Input: part model. Units: mm. Frame: model coordinates. A direction names the side the tool comes from. Round coordinates to 2 decimals unless told otherwise and drop trailing zeros. Loops run counter-clockwise (first coordinate to the right, second up) from the corner with the lowest first, then second, coordinate; pieces in that order, holes last. Notation, with made-up numbers: (87.25, 82) - (143.25, 82) arc R20 ccw to (143.25, 108) - close; hole circle Ø3 at (72, 65). An arc over 180 degrees is marked (long way). Write each question's results on one line, items separated by ' | '.
from build123d import *

# Parameters (mm, degrees)
SKETCH1_R           = 79.375
BOSS_EXTRUDE1_DEPTH = 25.4
SKETCH2_R           = 28.575
BOSS_EXTRUDE2_DEPTH = 3.175
SKETCH3_R           = 9.525
CUT_EXTRUDE1_DEPTH  = 19.05


with BuildPart() as part:
    # Sketch1 → Boss-Extrude1 (new body)
    with BuildSketch(Plane(origin=(0, 0, 0), x_dir=(1, 0, 0), z_dir=(0, 1, 0))):
        with Locations(Location((0, 0, 0), (0, 0, 270))):
            Circle(SKETCH1_R)
        with BuildLine():
            ThreePointArc((12.296722124, 3.175), (11.733270063, 4.860079591), (10.940159631, 6.45003157))
            Line((10.940159631, 6.45003157), (56.079808271, 51.589680211))
            ThreePointArc((56.079808271, 51.589680211), (70.399620377, 29.160477546), (76.133825433, 3.175))
            Line((76.133825433, 3.175), (12.296722124, 3.175))
        make_face(mode=Mode.SUBTRACT)
        with BuildLine():
            Line((51.589680211, 56.079808271), (6.45003157, 10.940159631))
            ThreePointArc((6.45003157, 10.940159631), (4.860079591, 11.733270063), (3.175, 12.296722124))
            Line((3.175, 12.296722124), (3.175, 76.133825433))
            ThreePointArc((3.175, 76.133825433), (29.160477546, 70.399620377), (51.589680211, 56.079808271))
        make_face(mode=Mode.SUBTRACT)
        with BuildLine():
            Line((-3.175, 76.133825433), (-3.175, 12.296722124))
            ThreePointArc((-3.175, 12.296722124), (-4.860079591, 11.733270063), (-6.45003157, 10.940159631))
            Line((-6.45003157, 10.940159631), (-51.589680211, 56.079808271))
            ThreePointArc((-51.589680211, 56.079808271), (-29.160477546, 70.399620377), (-3.175, 76.133825433))
        make_face(mode=Mode.SUBTRACT)
        with BuildLine():
            Line((-56.079808271, 51.589680211), (-10.940159631, 6.45003157))
            ThreePointArc((-10.940159631, 6.45003157), (-11.733270063, 4.860079591), (-12.296722124, 3.175))
            Line((-12.296722124, 3.175), (-76.133825433, 3.175))
            ThreePointArc((-76.133825433, 3.175), (-70.399620377, 29.160477546), (-56.079808271, 51.589680211))
        make_face(mode=Mode.SUBTRACT)
        with BuildLine():
            Line((-76.133825433, -3.175), (-12.296722124, -3.175))
            ThreePointArc((-12.296722124, -3.175), (-11.733270063, -4.860079591), (-10.940159631, -6.45003157))
            Line((-10.940159631, -6.45003157), (-56.079808271, -51.589680211))
            ThreePointArc((-56.079808271, -51.589680211), (-70.399620377, -29.160477546), (-76.133825433, -3.175))
        make_face(mode=Mode.SUBTRACT)
        with BuildLine():
            Line((-51.589680211, -56.079808271), (-6.45003157, -10.940159631))
            ThreePointArc((-6.45003157, -10.940159631), (-4.860079591, -11.733270063), (-3.175, -12.296722124))
            Line((-3.175, -12.296722124), (-3.175, -76.133825433))
            ThreePointArc((-3.175, -76.133825433), (-29.160477546, -70.399620377), (-51.589680211, -56.079808271))
        make_face(mode=Mode.SUBTRACT)
        with BuildLine():
            Line((3.175, -76.133825433), (3.175, -12.296722124))
            ThreePointArc((3.175, -12.296722124), (4.860079591, -11.733270063), (6.45003157, -10.940159631))
            Line((6.45003157, -10.940159631), (51.589680211, -56.079808271))
            ThreePointArc((51.589680211, -56.079808271), (29.160477546, -70.399620377), (3.175, -76.133825433))
        make_face(mode=Mode.SUBTRACT)
        with BuildLine():
            Line((56.079808271, -51.589680211), (10.940159631, -6.45003157))
            ThreePointArc((10.940159631, -6.45003157), (11.733270063, -4.860079591), (12.296722124, -3.175))
            Line((12.296722124, -3.175), (76.133825433, -3.175))
            ThreePointArc((76.133825433, -3.175), (70.399620377, -29.160477546), (56.079808271, -51.589680211))
        make_face(mode=Mode.SUBTRACT)
    extrude(amount=BOSS_EXTRUDE1_DEPTH)

    # Sketch2 → Boss-Extrude2 (add)
    with BuildSketch(Plane.XZ):
        Circle(SKETCH2_R)
    extrude(amount=-BOSS_EXTRUDE2_DEPTH)

    # Sketch3 → Cut-Extrude1 (cut)
    with BuildSketch(Plane.XZ):
        with Locations(Location((0, 0, 0), (0, 0, 270))):
            Circle(SKETCH3_R)
    extrude(amount=-CUT_EXTRUDE1_DEPTH, mode=Mode.SUBTRACT)


solid = part.part
1. Mould query, pull axis Z, two halves, no side actions, for faces 1 (the flat face through (9, 3.175, -20)), 2 (the flat face through (-17, 0, -1)). Classes: pulls with the +Z half, pulls with the -Z half, needs draft (parallel to the pull), parting line crosses it, or undercut.
Answer:
face 1: undercut | face 2: needs draft
2. Section query C-C, the plane x = -32. Output: boundary loops of the cut face in (y, z) (3 decimals), plus the area to 3 significant figures.
Answer:
outline: (0, -72.639) - (25.4, -72.639) - (25.4, -69.155) - (0, -69.155) - close; (0, -36.49) - (25.4, -36.49) - (25.4, -27.51) - (0, -27.51) - close; (0, -3.175) - (25.4, -3.175) - (25.4, 3.175) - (0, 3.175) - close; (0, 27.51) - (25.4, 27.51) - (25.4, 36.49) - (0, 36.49) - close; (0, 69.155) - (25.4, 69.155) - (25.4, 72.639) - (0, 72.639) - close | area: 794 mm^2
3. Section query B-B, the plane z = 48. Output: boundary loops of the cut face in (x, y) (3 decimals), plus the area to 3 significant figures.
Answer:
outline: (-63.217, 0) - (-59.181, 0) - (-59.181, 25.4) - (-63.217, 25.4) - close; (-52.49, 0) - (-43.51, 0) - (-43.51, 25.4) - (-52.49, 25.4) - close; (-3.175, 0) - (3.175, 0) - (3.175, 25.4) - (-3.175, 25.4) - close; (43.51, 0) - (52.49, 0) - (52.49, 25.4) - (43.51, 25.4) - close; (59.181, 0) - (63.217, 0) - (63.217, 25.4) - (59.181, 25.4) - close | area: 822 mm^2
4. Line query: line 1 (Z direction, x = 5.5, y = 20.75); line 2 (X direction, y = 7.25, z = 0) (3 decimals); line 3 (X direction, y = 19.5, z = 55) (3 decimals). Output: solid intervals per line, ascending. Write a range as [from, to].
Answer:
line 1: [-79.18, -76], [-11.45, 11.45], [76, 79.18] | line 2: [-79.375, -9.525], [9.525, 79.375] | line 3: [-57.231, -50.51], [-3.175, 3.175], [50.51, 57.231]
5. Set-up query: faces 3 (the cylindrical face through (-11.039, 1.565, -26.357)), 4 (the cylindrical face through (-5.796, 9.392, 7.559)), 5 (the flat face through (33.83, 12.52, 29.34)). Return all of +Z, -Z, +X, -X, +Y, -Y with unobstructed straight access to the full face (end or side cutting, diameter ignored); none if empty.
Answer:
face 3: +Y, -Y | face 4: -Y | face 5: +Y
6. Contact query for flat-ended pins moving along their axis: pin 1 (1.5 mm diameter, centred on x = -41.5, y = 20, fed in from -Z); pin 2 (7.5 mm diameter, centred on y = 13.5, z = 48, fed in from +X); pin 3 (10 mm diameter, centred on x = 13.5, z = -34.5, fed in from +Y); pin 4 (4 mm diameter, centred on y = 8, z = 13, fed in from -X). Output: stop coordinate, or through.
Answer:
pin 1: z = -68.12 | pin 2: x = 65.9 | pin 3: through | pin 4: x = -78.61
7. Section query A-A, the plane y = 11. Count the separate pieces of the cut face and the enclosed holes in it, plus the area to 3 significant figures.
Answer:
separate pieces: 1 | enclosed holes: 9 | area: 5,000 mm^2
